Read the model definition and answer for the solid it produces. Units are mm, in the model's axes. A direction names the side the tool comes from. Round coordinates to 2 decimals unless told otherwise and drop trailing zeros. Write each loop counter-clockwise with the first axis right and the second up, starting at its lowest first coordinate (ties: lowest second). Pieces come first, ordered by that corner, then holes.
from build123d import *

# Parameters (mm, degrees)
SKETCH1_R           = 60
BOSS_EXTRUDE1_DEPTH = 130
FILLET1_R           = 10
SKETCH2_R           = 55
BOSS_EXTRUDE2_DEPTH = 150
SKETCH3_R           = 42.5
CUT_EXTRUDE1_DEPTH  = 150


with BuildPart() as part:
    # Sketch1 → Boss-Extrude1 (new body)
    with BuildSketch(Plane(origin=(0, 0, 0), x_dir=(1, 0, 0), z_dir=(0, 1, 0))):
        Circle(SKETCH1_R)
    extrude(amount=BOSS_EXTRUDE1_DEPTH)

    # Fillet1
    fillet1_edges = [part.edges().sort_by_distance(p)[0] for p in [
        (-60, 130, 0),
    ]]
    fillet(fillet1_edges, radius=FILLET1_R)

    # Sketch2 → Boss-Extrude2 (add)
    with BuildSketch(Plane(origin=(0, 0, 0), x_dir=(0, 0, -1), z_dir=(1, 0, 0))):
        with Locations((0, 60)):
            Circle(SKETCH2_R)
    extrude(amount=BOSS_EXTRUDE2_DEPTH)

    # Sketch3 → Cut-Extrude1 (cut)
    with BuildSketch(Plane(origin=(0, 0, 0), x_dir=(0, 0, -1), z_dir=(1, 0, 0))):
        with Locations((0, 60)):
            Circle(SKETCH3_R)
    extrude(amount=CUT_EXTRUDE1_DEPTH, mode=Mode.SUBTRACT)


solid = part.part
Q1. Flat-ended cylindrical pins translate along their axes: pin 1 Ø3 at (x, y) = (82, 29) entering from -Z; pin 2 Ø1.5 at (y, z) = (45, 37.5) entering from +X; pin 3 Ø8 at (x, y) = (41.5, 35.5) entering from +Z. Find the tip coordinate at first contact, or state that the pin passes through.
Verdict:
pin 1: stops at z = -46.42
pin 2: stops at x = 0
pin 3: stops at z = 51.04
Q2. Section B-B (z = 0) is taken. Determine the outline of the cut face in (x, y).
Verdict:
outline: (-60, 0) - (60, 0) - (60, 5) - (150, 5) - (150, 17.5) - (0, 17.5) - (0, 102.5) - (150, 102.5) - (150, 115) - (60, 115) - (60, 120) arc R10 ccw to (50, 130) - (-50, 130) arc R10 ccw to (-60, 120) - close
Q3. Section D-D (y = 38) is taken. Determine the outline of the cut face in (x, z).
Verdict:
outline: (0, -36.36) - (0, 36.36) - (150, 36.36) - (150, 50.41) - (32.54, 50.41) arc R60 ccw (long way) to (32.54, -50.41) - (150, -50.41) - (150, -36.36) - close
Q4. Which of the six approach directions +Z, -Z, +X, -X, +Y, -Y give full straight-line access (tool end or side, diameter ignored) to faces 5 (the cylindrical face through (100.11, 38.935, -50.806)), 6 (the flat face through (-1, 130, -1))?
Verdict:
face 5: +X
face 6: +Z, -Z, +X, -X, +Y
Q5. Determine the mould class of faces 1 (the flat face through (0, 61, 1)), 2 (the cylindrical face through (73.95, 95.836, -22.848)), 3 (the flat face through (150, 27.7, -28.3)), 4 (the cylindrical face through (-59.94, 59.16, -2.64)) for opening direction Z: pulls with the +Z half, pulls with the -Z half, needs draft (parallel to the pull), parting line crosses it, or undercut.
Verdict:
face 1: undercut
face 2: undercut
face 3: needs draft
face 4: parting line crosses it
Q6. Section C-C (x = 124) is taken. Determine the outline of the cut face in (y, z), then the cut area to 3 significant figures.
Verdict:
outline: circle Ø110 at (60, 0); hole circle Ø85 at (60, 0)
area: 3,830 mm2
Q7. Section A-A (y = 60) is taken. Determine the outline of the cut face in (x, z).
Verdict:
outline: (0, -42.5) - (0, 42.5) - (150, 42.5) - (150, 55) - (23.98, 55) arc R60 ccw (long way) to (23.98, -55) - (150, -55) - (150, -42.5) - close
Q8. Straight lines are drawn through the part: probe 1 along Y at (x, z) = (83, 0); probe 2 along Z at (x, y) = (101, 77); probe 3 along Z at (x, y) = (103, 75.5). For each, find the intervals that lie inside material, in ascending order.
Verdict:
probe 1: y = 5 to 17.5, 102.5 to 115
probe 2: z = -52.31 to -38.95, 38.95 to 52.31
probe 3: z = -52.77 to -39.57, 39.57 to 52.77
